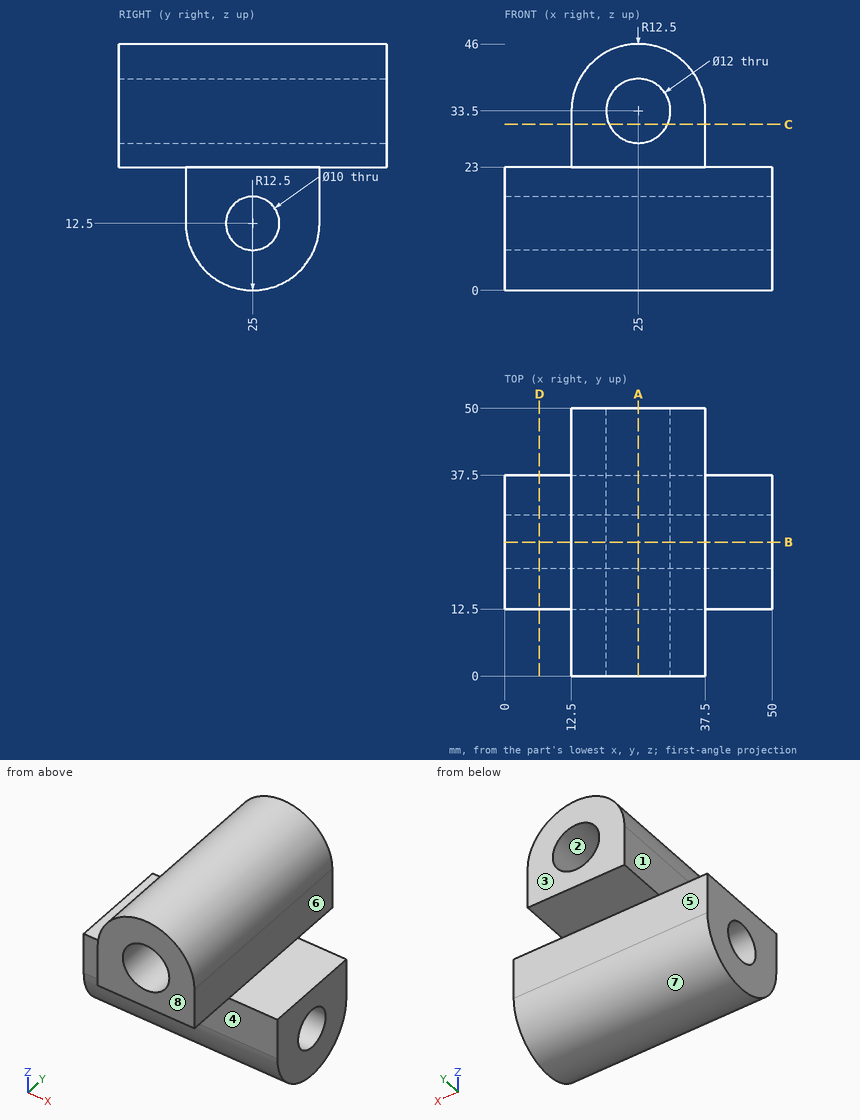
Check sheet for the drawn part. Datum: minimum x, y, z corner. Units: mm. A direction names the side the tool comes from. Give positions to 0.01 mm unless a question says otherwise; leave off trailing zeros. Write each loop counter-clockwise with the first axis right and the second up, starting at its lowest first coordinate (ties: lowest second). Pieces come first, ordered by that corner, then holes. Notation, with made-up numbers: M 79,26.25 L 99,26.25 A15 cw 99,39.25 Z; hole C 47,23.5 d3. An arc over 180 degrees is marked long. One line per question, with ' | ' between items.
1) Mould release check, pull along X, two halves, no side actions. Record for the marked faces 1, 2 and 3: released by +X, released by -X, zero draft, split by the parting line, or undercut.
Result:
face 1: released by -X | face 2: undercut | face 3: zero draft
2) Set-up check for the marked faces 4, 5, 6, 7 and 8: record each of +Z, -Z, +X, -X, +Y, -Y from which the full face is reachable in a straight line by a thin tool's end or side.
Result:
face 4: -Z, +X, -X, -Y | face 5: -Z, +X, -X, +Y | face 6: +Z, +X, +Y, -Y | face 7: -Z, +X, -X | face 8: +Z, -Z, +X, -X, -Y
3) Section check C-C on z = 31. Enter the section's corners in (x, y), plus the area to 3 significant figures.
Result:
outline: M 12.5,0 L 19.55,0 L 19.55,50 L 12.5,50 Z; M 30.45,0 L 37.5,0 L 37.5,50 L 30.45,50 Z | area: 705 mm2
4) Section check A-A on x = 25. Enter the section's corners in (y, z).
Result:
outline: M 0,23 L 12.5,23 L 12.5,12.5 A12.5 ccw 37.5,12.5 L 37.5,23 L 50,23 L 50,27.5 L 0,27.5 Z; M 0,39.5 L 50,39.5 L 50,46 L 0,46 Z; hole C 25,12.5 d10
5) Thickness scan on line 1 along Z through (x, y) = (22, 26.5); line 2 along Z through (x, y) = (27.5, 25); line 3 along Z through (x, y) = (25, 11). Record the ranges inside material, lowest first. Write a range as [from, to].
Result:
line 1: z = [0.09, 7.73], [17.27, 28.3], [38.7, 45.63] | line 2: z = [0, 7.5], [17.5, 28.05], [38.95, 45.75] | line 3: z = [23, 27.5], [39.5, 46]
6) Gauge pin test, flat ends, axial feed: pin 1 Ø5 at (x, z) = (27.5, 19) entering from -Y; pin 2 Ø12 at (x, y) = (41, 20) entering from +Z; pin 3 Ø8.5 at (x, z) = (20, 17) entering from +Y. Record the tip position at first contact, or that the pin passes through.
Result:
pin 1: stops at y = 12.5 | pin 2: stops at z = 41 | pin 3: stops at y = 37.5
7) Section check B-B on y = 25. Enter the section's corners in (x, z).
Result:
outline: M 0,0 L 50,0 L 50,7.5 L 0,7.5 Z; M 0,17.5 L 50,17.5 L 50,23 L 37.5,23 L 37.5,33.5 A12.5 ccw 12.5,33.5 L 12.5,23 L 0,23 Z; hole C 25,33.5 d12
8) Section check D-D on x = 6.5. Enter the section's corners in (y, z), plus the area to 3 significant figures.
Result:
outline: M 12.5,12.5 A12.5 ccw 37.5,12.5 L 37.5,23 L 12.5,23 Z; hole C 25,12.5 d10 | area: 429 mm2
